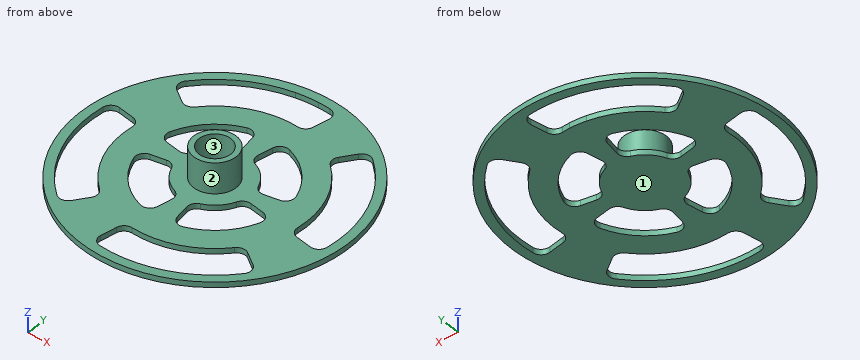
Autodesk Fusion 360 part; units mm, degrees
sketch "Sketch1" plane through (0, 0, 0) normal (0, 0, 1) x (1, 0, 0)
  circle A0 centre (0, 0) radius 75
  circle A1 centre (0, 0) radius 46
  circle A2 centre (0, 0) radius 43
  circle A3 centre (0, 0) radius 11.9
  circle A4 centre (0, 0) radius 8.9
  line L0 (0, 90) -> (0, -90)
  line L1 (12.1554, 68.9365) -> (13.0236, 73.8606)
  line L2 (8.8561, 50.2252) -> (12.1554, 68.9365)
  line L3 (-12.1554, 68.9365) -> (-13.0236, 73.8606)
  line L4 (-8.8561, 50.2252) -> (-12.1554, 68.9365)
  arc A5 (-8.8561, 50.2252) -> (8.8561, 50.2252) centre (0, 0) ccw
  arc A6 (0, 51) -> (-8.8561, 50.2252) centre (0, 0) ccw
  arc A7 (8.8561, 50.2252) -> (0, 51) centre (0, 0) ccw
  arc A8 (-12.1554, 68.9365) -> (12.1554, 68.9365) centre (0, 0) ccw
  arc A9 (12.1554, 68.9365) -> (0, 70) centre (0, 0) ccw
  arc A10 (0, 70) -> (-12.1554, 68.9365) centre (0, 0) ccw
  arc A11 (-6.5986, 37.4227) -> (6.5986, 37.4227) centre (0, 0) ccw
  arc A12 (6.5986, 37.4227) -> (0, 38) centre (0, 0) ccw
  arc A13 (0, 38) -> (-6.5986, 37.4227) centre (0, 0) ccw
  line L5 (0, 0) -> (3.473, 19.6962)
  line L6 (6.5986, 37.4227) -> (8.8561, 50.2252)
  line L7 (3.473, 19.6962) -> (6.5986, 37.4227)
  line L8 (0, 0) -> (-3.473, 19.6962)
  line L9 (-6.5986, 37.4227) -> (-8.8561, 50.2252)
  line L10 (-3.473, 19.6962) -> (-6.5986, 37.4227)
  arc A14 (-3.473, 19.6962) -> (3.473, 19.6962) centre (0, 0) ccw
  arc A15 (0, 20) -> (-3.473, 19.6962) centre (0, 0) ccw
  arc A16 (3.473, 19.6962) -> (0, 20) centre (0, 0) ccw
  arc A17 (-40.1504, 57.3406) -> (-49.4975, 49.4975) centre (0, 0) ccw
  arc A18 (-49.4975, 49.4975) -> (-57.3406, 40.1504) centre (0, 0) ccw
  line L11 (-29.2524, 41.7768) -> (-40.1504, 57.3406)
  arc A19 (-29.2524, 41.7768) -> (-36.0624, 36.0624) centre (0, 0) ccw
  arc A20 (-36.0624, 36.0624) -> (-41.7768, 29.2524) centre (0, 0) ccw
  line L12 (-41.7768, 29.2524) -> (-57.3406, 40.1504)
  arc A21 (-21.7959, 31.1278) -> (-26.8701, 26.8701) centre (0, 0) ccw
  line L13 (-11.4715, 16.383) -> (-21.7959, 31.1278)
  arc A22 (-11.4715, 16.383) -> (-14.1421, 14.1421) centre (0, 0) ccw
  arc A23 (-14.1421, 14.1421) -> (-16.383, 11.4715) centre (0, 0) ccw
  line L14 (-16.383, 11.4715) -> (-31.1278, 21.7959)
  arc A24 (-26.8701, 26.8701) -> (-31.1278, 21.7959) centre (0, 0) ccw
  arc A25 (-68.9365, 12.1554) -> (-70, 0) centre (0, 0) ccw
  arc A26 (-70, 0) -> (-68.9365, -12.1554) centre (0, 0) ccw
  line L15 (-50.2252, 8.8561) -> (-68.9365, 12.1554)
  arc A27 (-50.2252, 8.8561) -> (-51, 0) centre (0, 0) ccw
  arc A28 (-51, 0) -> (-50.2252, -8.8561) centre (0, 0) ccw
  line L16 (-50.2252, -8.8561) -> (-68.9365, -12.1554)
  arc A29 (-37.4227, 6.5986) -> (-38, 0) centre (0, 0) ccw
  line L17 (-19.6962, 3.473) -> (-37.4227, 6.5986)
  arc A30 (-19.6962, 3.473) -> (-20, 0) centre (0, 0) ccw
  arc A31 (-20, 0) -> (-19.6962, -3.473) centre (0, 0) ccw
  line L18 (-19.6962, -3.473) -> (-37.4227, -6.5986)
  arc A32 (-38, 0) -> (-37.4227, -6.5986) centre (0, 0) ccw
  arc A33 (-57.3406, -40.1504) -> (-49.4975, -49.4975) centre (0, 0) ccw
  arc A34 (-49.4975, -49.4975) -> (-40.1504, -57.3406) centre (0, 0) ccw
  line L19 (-41.7768, -29.2524) -> (-57.3406, -40.1504)
  arc A35 (-41.7768, -29.2524) -> (-36.0624, -36.0624) centre (0, 0) ccw
  arc A36 (-36.0624, -36.0624) -> (-29.2524, -41.7768) centre (0, 0) ccw
  line L20 (-29.2524, -41.7768) -> (-40.1504, -57.3406)
  arc A37 (-31.1278, -21.7959) -> (-26.8701, -26.8701) centre (0, 0) ccw
  line L21 (-16.383, -11.4715) -> (-31.1278, -21.7959)
  arc A38 (-16.383, -11.4715) -> (-14.1421, -14.1421) centre (0, 0) ccw
  arc A39 (-14.1421, -14.1421) -> (-11.4715, -16.383) centre (0, 0) ccw
  line L22 (-11.4715, -16.383) -> (-21.7959, -31.1278)
  arc A40 (-26.8701, -26.8701) -> (-21.7959, -31.1278) centre (0, 0) ccw
  arc A41 (-12.1554, -68.9365) -> (0, -70) centre (0, 0) ccw
  arc A42 (0, -70) -> (12.1554, -68.9365) centre (0, 0) ccw
  line L23 (-8.8561, -50.2252) -> (-12.1554, -68.9365)
  arc A43 (-8.8561, -50.2252) -> (0, -51) centre (0, 0) ccw
  arc A44 (0, -51) -> (8.8561, -50.2252) centre (0, 0) ccw
  line L24 (8.8561, -50.2252) -> (12.1554, -68.9365)
  arc A45 (-6.5986, -37.4227) -> (0, -38) centre (0, 0) ccw
  line L25 (-3.473, -19.6962) -> (-6.5986, -37.4227)
  arc A46 (-3.473, -19.6962) -> (0, -20) centre (0, 0) ccw
  arc A47 (0, -20) -> (3.473, -19.6962) centre (0, 0) ccw
  line L26 (3.473, -19.6962) -> (6.5986, -37.4227)
  arc A48 (0, -38) -> (6.5986, -37.4227) centre (0, 0) ccw
  arc A49 (40.1504, -57.3406) -> (49.4975, -49.4975) centre (0, 0) ccw
  arc A50 (49.4975, -49.4975) -> (57.3406, -40.1504) centre (0, 0) ccw
  line L27 (29.2524, -41.7768) -> (40.1504, -57.3406)
  arc A51 (29.2524, -41.7768) -> (36.0624, -36.0624) centre (0, 0) ccw
  arc A52 (36.0624, -36.0624) -> (41.7768, -29.2524) centre (0, 0) ccw
  line L28 (41.7768, -29.2524) -> (57.3406, -40.1504)
  arc A53 (21.7959, -31.1278) -> (26.8701, -26.8701) centre (0, 0) ccw
  line L29 (11.4715, -16.383) -> (21.7959, -31.1278)
  arc A54 (11.4715, -16.383) -> (14.1421, -14.1421) centre (0, 0) ccw
  arc A55 (14.1421, -14.1421) -> (16.383, -11.4715) centre (0, 0) ccw
  line L30 (16.383, -11.4715) -> (31.1278, -21.7959)
  arc A56 (26.8701, -26.8701) -> (31.1278, -21.7959) centre (0, 0) ccw
  arc A57 (68.9365, -12.1554) -> (70, 0) centre (0, 0) ccw
  arc A58 (70, 0) -> (68.9365, 12.1554) centre (0, 0) ccw
  line L31 (50.2252, -8.8561) -> (68.9365, -12.1554)
  arc A59 (50.2252, -8.8561) -> (51, 0) centre (0, 0) ccw
  arc A60 (51, 0) -> (50.2252, 8.8561) centre (0, 0) ccw
  line L32 (50.2252, 8.8561) -> (68.9365, 12.1554)
  arc A61 (37.4227, -6.5986) -> (38, 0) centre (0, 0) ccw
  line L33 (19.6962, -3.473) -> (37.4227, -6.5986)
  arc A62 (19.6962, -3.473) -> (20, 0) centre (0, 0) ccw
  arc A63 (20, 0) -> (19.6962, 3.473) centre (0, 0) ccw
  line L34 (19.6962, 3.473) -> (37.4227, 6.5986)
  arc A64 (38, 0) -> (37.4227, 6.5986) centre (0, 0) ccw
  arc A65 (57.3406, 40.1504) -> (49.4975, 49.4975) centre (0, 0) ccw
  arc A66 (49.4975, 49.4975) -> (40.1504, 57.3406) centre (0, 0) ccw
  line L35 (41.7768, 29.2524) -> (57.3406, 40.1504)
  arc A67 (41.7768, 29.2524) -> (36.0624, 36.0624) centre (0, 0) ccw
  arc A68 (36.0624, 36.0624) -> (29.2524, 41.7768) centre (0, 0) ccw
  line L36 (29.2524, 41.7768) -> (40.1504, 57.3406)
  arc A69 (31.1278, 21.7959) -> (26.8701, 26.8701) centre (0, 0) ccw
  line L37 (16.383, 11.4715) -> (31.1278, 21.7959)
  arc A70 (16.383, 11.4715) -> (14.1421, 14.1421) centre (0, 0) ccw
  arc A71 (14.1421, 14.1421) -> (11.4715, 16.383) centre (0, 0) ccw
  line L38 (11.4715, 16.383) -> (21.7959, 31.1278)
  arc A72 (26.8701, 26.8701) -> (21.7959, 31.1278) centre (0, 0) ccw
  dimension "d1" = 150
  dimension "d2" = -29
  dimension "d3" = -3
  dimension "d12" = 23.8
  dimension "d13" = -3
  dimension "d20" = 10
  dimension "d21" = 20
  dimension "d23" = 360
extrude "Extrude1" add sketch "Sketch1" along normal blind 3
extrude "Extrude3" add sketch "Sketch1" along normal blind 20 contours A3 A4 L0 L5 | A3 A4 L0 L5 | A3 A4 L0 L8 | A3 A4 L0 L8
extrude "Extrude4" cut sketch "Sketch1" along normal up to surface (3 mm away) contours L0 L2 A7 A9 | L0 A5 A8 A41 L23 A43 | L0 A5 A8 A42 A44 L24 | L0 L4 A6 A10 | A5 A8 A65 A66 L35 A67 A68 L36 | L4 A5 A8 L11 | A5 A8 L24 L27 | A5 A8 A17 A18 L11 A19 A20 L12 | A5 A8 A33 A34 L19 A35 A36 L20 | A5 A8 A49 A50 L27 A51 A52 L28 | A5 A8 L32 L35 | A5 A8 A57 A58 L31 A59 A60 L32 | A5 A8 L16 L19 | A5 A8 A25 A26 L15 A27 A28 L16
fillet "Fillet5" radius 5 16 edges at (-68.9365, 12.1554, 1.5) (-50.2252, 8.8561, 1.5) (-40.1504, -57.3406, 1.5) (-29.2524, -41.7768, 1.5) (-12.1554, -68.9365, 1.5) (-8.8561, -50.2252, 1.5) (57.3406, -40.1504, 1.5) (41.7768, -29.2524, 1.5) (68.9365, -12.1554, 1.5) (50.2252, -8.8561, 1.5) (40.1504, 57.3406, 1.5) (29.2524, 41.7768, 1.5) (8.8561, 50.2252, 1.5) (12.1554, 68.9365, 1.5) (-57.3406, 40.1504, 1.5) (-41.7768, 29.2524, 1.5)
extrude "Extrude5" cut sketch "Sketch1" along normal up to surface (3 mm away) contours A11 L7 A14 L38 | A11 A14 A69 L37 A70 A71 L38 A72 | A11 L10 A14 L13 | A11 A14 L22 L25 | A11 A14 L26 L29 | A11 A14 A21 L13 A22 A23 L14 A24 | A11 A14 A37 L21 A38 A39 L22 A40 | A11 A14 A53 L29 A54 A55 L30 A56 | A11 A14 L34 L37 | A11 A14 L14 L17 | A11 A14 L18 L21 | A11 A14 L30 L33
fillet "Fillet6" radius 5 16 edges at (-6.5986, 37.4227, 1.5) (-3.473, 19.6962, 1.5) (-37.4227, 6.5986, 1.5) (-19.6962, 3.473, 1.5) (-37.4227, -6.5986, 1.5) (-19.6962, -3.473, 1.5) (-6.5986, -37.4227, 1.5) (-3.473, -19.6962, 1.5) (6.5986, -37.4227, 1.5) (3.473, -19.6962, 1.5) (19.6962, -3.473, 1.5) (37.4227, -6.5986, 1.5) (37.4227, 6.5986, 1.5) (19.6962, 3.473, 1.5) (6.5986, 37.4227, 1.5) (3.473, 19.6962, 1.5)
Read the model definition and answer for the solid it produces. Units are mm, in the model's axes. Face numbers are marked on the shaded views. Coordinates: 2 decimals unless noted, no trailing zeros. Order: outer loops, then holes, each group sorted by start corner. A loop starts at its lowest first (then second) coordinate and runs counter-clockwise, first axis right, second up. Notation, with made-up numbers: (79, 39.25) - (117, 39.25) arc R18 cw to (117, 52.25) - close; hole circle Ø4 at (-27.5, 68.25). An arc over 180 degrees is marked (long way). Answer as a JSON object with one key per item and string values. Group by question number.
Item 1: Section B-B (x = 66) is taken. Give the vertices of the cut face in (y, z), plus the area to 3 significant figures.
Item 2: Consider probe 1 along Y at (x, z) = (0, 11.5); probe 2 along X at (y, z) = (26.5, 2.5). Determine where each line is inside the solid, lowest interval first. Write a range as from..to.
Item 3: Section D-D (y = -60) is taken. Give the vertices of the cut face in (x, z).
Item 4: Section A-A (y = 0) is taken. Give the vertices of the cut face in (x, z).
Item 5: The mould has two halves that part along Y. Classify the marked faces 1, 2 and 3: +Y half, -Y half, draft (parallel to the pull), parting line (faces both ways), or undercut.
Item 6: Flat-ended cylindrical pins translate along their axes: P1, Ø5.5, axis at x = 0.5, y = 4.5, coming from the +Z side; P2, Ø1.5, axis at x = -36.5, y = 26, coming from the -Z side; P3, Ø10, axis at x = -23, z = 11.5, coming from the +Y side; P4, Ø2, axis at x = 9, z = 6.5, coming from the +Y side. Find the tip coordinate at first contact, or state that the pin passes through.
Item 7: Section C-C (z = 7.5) is taken. Give the vertices of the cut face in (x, y).
Results are:
{
 "1": {"outline": "(-35.62, 0) - (-11.16, 0) - (-11.16, 3) - (-35.62, 3) - close; (23.32, 0) - (35.62, 0) - (35.62, 3) - (23.32, 3) - close", "area": "110 mm^2"},
 "2": {"probe 1": "y = -11.9..-8.9, 8.9..11.9", "probe 2": "x = -70.16..-27.24, -4.67..4.67, 27.24..43.57, 64.79..70.16"},
 "3": {"outline": "(-45, 0) - (-10.58, 0) - (-10.58, 3) - (-45, 3) - close; (36.06, 0) - (45, 0) - (45, 3) - (36.06, 3) - close"},
 "4": {"outline": "(-75, 0) - (-70, 0) - (-70, 3) - (-75, 3) - close; (-51, 0) - (51, 0) - (51, 3) - (11.9, 3) - (11.9, 20) - (8.9, 20) - (8.9, 3) - (-8.9, 3) - (-8.9, 20) - (-11.9, 20) - (-11.9, 3) - (-51, 3) - close; (70, 0) - (75, 0) - (75, 3) - (70, 3) - close"},
 "5": {"face 1": "draft", "face 2": "parting line", "face 3": "undercut"},
 "6": {"P1": "stops at z = 3", "P2": "stops at z = 0", "P3": "passes through", "P4": "stops at y = 8.81"},
 "7": {"outline": "circle Ø23.8 at (0, 0); hole circle Ø17.8 at (0, 0)"}
}
